Read the model definition and answer for the solid it produces. Units are mm, in the model's axes. Face numbers are marked on the shaded views. A direction names the side the tool comes from. Round coordinates to 2 decimals unless told otherwise and drop trailing zeros. Order: outer loops, then holes, each group sorted by start corner. A loop starts at its lowest first (then second) coordinate and runs counter-clockwise, first axis right, second up. Notation, with made-up numbers: (48.25, 59) - (92.25, 59) arc R6 cw to (92.25, 63) - close; hole circle Ø3 at (19.5, -7). An arc over 180 degrees is marked (long way). Put each result on its own line as item: value. Start each with the question number.
Q1. Find the intervals of material crossed by line 1 along Z through (x, y) = (0.5, -1.25); line 2 along Z through (x, y) = (3, -0.5); line 3 along Y through (x, z) = (-1.25, 15.75), in increasing order. Write a range as from..to.
Q2. Section A-A on z = 20.5 is taken. Give the vertices of the cut face in (x, y).
Q3. Which of the six approach directions +Z, -Z, +X, -X, +Y, -Y give full straight-line access (tool end or side, diameter ignored) to the marked faces 4, 5 and 6?
Q4. Section C-C on z = 2.5 is taken. Give the vertices of the cut face in (x, y), then the cut area to 3 significant figures.
Q5. Section B-B on y = 0 is taken. Give the vertices of the cut face in (x, z).
Q6. For a pull along Y with two mould halves and no side action, classify the marked faces 1, 2 and 3 as pulls with the +Y half, pulls with the -Y half, needs draft (parallel to the pull), parting line crosses it, or undercut.
Q7. Each of these flat-tipped pins is pushed along its axis until it touches: pin 1 Ø5 at (y, z) = (3.5, 5.5) entering from +X; pin 2 Ø2 at (y, z) = (-1.5, 3) entering from +X; pin 3 Ø1.5 at (x, y) = (-3.5, 3.5) entering from -Z. Where does it stop, or does it pass through?
from build123d import *

# Parameters (mm, degrees)
FILLET_R     = 1
POCKET_DEPTH = 3


with BuildPart() as part:
    # Sketch → Revolution (revolve)
    with BuildSketch(Plane.XZ):
        Polygon((0, 0), (0, 22), (5, 22), (5, 16), (3, 16), (3, 12), (3, 1), (2, 0), align=None)
    revolve(axis=Axis((0, 0, 0), (0, 0, 1)))

    # Fillet
    fillet_edges = [part.edges().sort_by_distance(p)[0] for p in [
        (-5, 0, 22),
    ]]
    fillet(fillet_edges, radius=FILLET_R)

    # Sketch001 (on DatumPlane) → Pocket (cut)
    with BuildSketch(Plane.XY.offset(22)):
        Polygon((2.5, 1.443376), (0, 2.886751), (-2.5, 1.443376), (-2.5, -1.443376), (0, -2.886751), (2.5, -1.443376), align=None)
    extrude(amount=-POCKET_DEPTH, mode=Mode.SUBTRACT)


solid = part.part
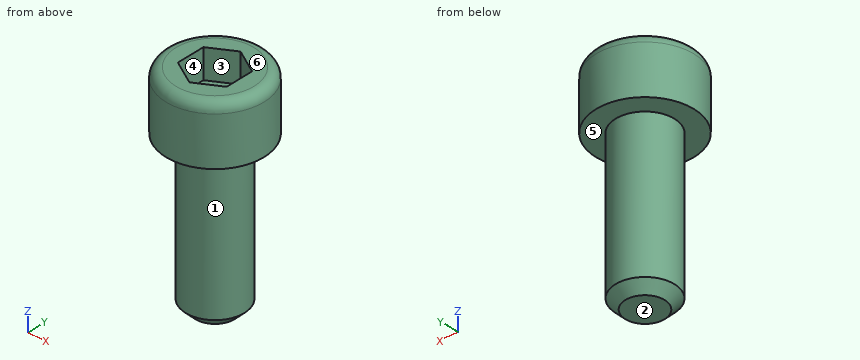
Findings:
1. line 1: 0..19
1. line 2: 16..22
1. line 3: -2.73..2.73
2. outline: circle Ø10 at (0, 0); hole (-2.5, -1.44) - (0, -2.89) - (2.5, -1.44) - (2.5, 1.44) - (0, 2.89) - (-2.5, 1.44) - close
3. face 4: +Z
3. face 5: -Z
3. face 6: +Z, +X, -X, +Y, -Y
4. outline: circle Ø6 at (0, 0)
4. area: 28.3 mm2
5. outline: (-5, 16) - (-3, 16) - (-3, 1) - (-2, 0) - (2, 0) - (3, 1) - (3, 16) - (5, 16) - (5, 21) arc R1 ccw to (4, 22) - (2.5, 22) - (2.5, 19) - (-2.5, 19) - (-2.5, 22) - (-4, 22) arc R1 ccw to (-5, 21) - close
6. face 1: parting line crosses it
6. face 2: needs draft
6. face 3: undercut
7. pin 1: x = 2.83
7. pin 2: x = 2.96
7. pin 3: z = 16
